Work out the finished part from the listing and answer in its coordinate system (mm). Face numbers are marked on the shaded views. A direction names the side the tool comes from. Round coordinates to 2 decimals unless told otherwise and drop trailing zeros. Write each loop counter-clockwise with the first axis right and the second up, starting at its lowest first coordinate (ties: lowest second). Pieces come first, ordered by that corner, then holes. Notation, with made-up numbers: M 29.25,75 L 44.25,75 A24 cw 44.25,95 Z; hole C 45,40 d1. An arc over 180 degrees is marked long. Answer in a Markdown table with one row per item.
```python
from build123d import *

# Parameters (mm, degrees)
CHAMFER1_SIZE = 1
CHAMFER2_SIZE = 1


with BuildPart() as part:
    # Sketch1 → Revolve1 (revolve)
    with BuildSketch(Plane(origin=(0, 0, 0), x_dir=(0, 0, -1), z_dir=(1, 0, 0))):
        Polygon((2.5, 9), (2.5, 0), (3.6, 0), (3.6, 8), (6, 8), (6, 9), align=None)
    revolve(axis=Axis((0, 0, 0), (0, 1, 0)))

    # Chamfer1
    chamfer1_edges = [part.edges().sort_by_distance(p)[0] for p in [
        (0, 8, 3.6),
    ]]
    chamfer(chamfer1_edges, length=CHAMFER1_SIZE)

    # Chamfer2
    chamfer2_edges = [part.edges().sort_by_distance(p)[0] for p in [
        (0, 9, 2.5),
    ]]
    chamfer(chamfer2_edges, length=CHAMFER2_SIZE)


solid = part.part
```
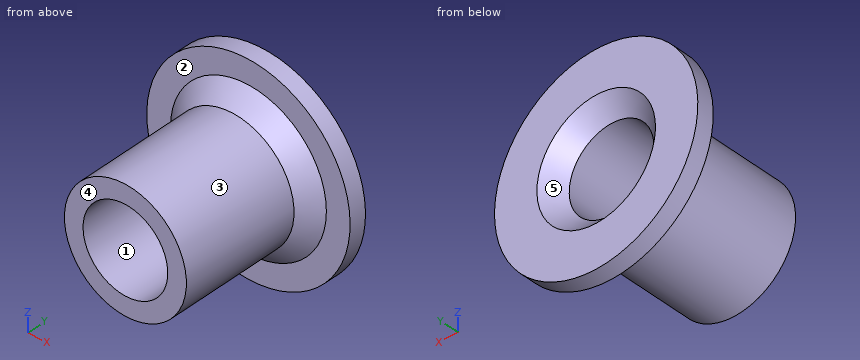
1. The part is cut by section B-B (z = 0). Determine the outline of the cut face in (x, y), plus the area to 3 significant figures.
Calculated:
| item | result |
|---|---|
| outline | M -6,8 L -4.6,8 L -3.6,7 L -3.6,0 L -2.5,0 L -2.5,8 L -3.5,9 L -6,9 Z; M 2.5,0 L 3.6,0 L 3.6,7 L 4.6,8 L 6,8 L 6,9 L 3.5,9 L 2.5,8 Z |
| area | 24.6 mm² |
2. Determine the mould class of the marked faces 3, 4 and 5 for opening direction X: released by +X, released by -X, zero draft, split by the parting line, or undercut.
Calculated:
| item | result |
|---|---|
| face 3 | split by the parting line |
| face 4 | zero draft |
| face 5 | undercut |
3. Consider line 1 along X through (y, z) = (4.5, 0); line 2 along Y through (x, z) = (5, 0.5). Determine where each line is inside the solid, lowest interval first. Write a range as from..to.
Calculated:
| item | result |
|---|---|
| line 1 | x = -3.6..-2.5, 2.5..3.6 |
| line 2 | y = 8..9 |
4. A tool of negligible diameter and unlimited length cuts with its end or side. For the marked faces 1 and 2, from which of +Z, -Z, +X, -X, +Y, -Y can it reach the whole face along a straight path? Write none if from no direction.
Calculated:
| item | result |
|---|---|
| face 1 | +Y, -Y |
| face 2 | -Y |
5. Given pin 1 (2 mm diameter, centred on y = 7.5, z = 2.5, fed in from -X); pin 2 (6 mm diameter, centred on x = 0, z = 0, fed in from +Y); pin 3 (4 mm diameter, centred on x = -4.5, y = 4, fed in from -Z), each flat-ended and moving along its own axis, determine where each tip first touches the part or whether it passes through.
Calculated:
| item | result |
|---|---|
| pin 1 | stops at x = -5.77 |
| pin 2 | stops at y = 8.5 |
| pin 3 | stops at z = -2.59 |
6. The part is cut by section C-C (y = 5). Determine the outline of the cut face in (x, z).
Calculated:
| item | result |
|---|---|
| outline | C 0,0 d7.2; hole C 0,0 d5 |
7. The part is cut by section A-A (x = 0). Determine the outline of the cut face in (y, z).
Calculated:
| item | result |
|---|---|
| outline | M 0,-3.6 L 7,-3.6 L 8,-4.6 L 8,-6 L 9,-6 L 9,-3.5 L 8,-2.5 L 0,-2.5 Z; M 0,2.5 L 8,2.5 L 9,3.5 L 9,6 L 8,6 L 8,4.6 L 7,3.6 L 0,3.6 Z |
8. The part is cut by section D-D (z = -5). Determine the outline of the cut face in (x, y).
Calculated:
| item | result |
|---|---|
| outline | M -3.32,8 L 3.32,8 L 3.32,9 L -3.32,9 Z |
